```python
from build123d import *

# Parameters (mm, degrees)
BOSS_EXTRUDE1_DEPTH = 10
BOSS_EXTRUDE2_DEPTH = 10
MIRROR1_START       = 20
MIRROR1_DEPTH       = 20
MIRROR1_START_2     = 30
MIRROR1_2_DEPTH     = 10
MIRROR1_3_DEPTH     = 10
FILLET1_R           = 2
FILLET2_R           = 1
SKETCH3_R           = 11
BOSS_EXTRUDE3_DEPTH = 2
SKETCH4_R           = 1.5
CUT_EXTRUDE1_DEPTH  = 4.5
SKETCH5_R           = 2.5
CUT_EXTRUDE3_DEPTH  = 52.521063654
CHAMFER3_SIZE       = 0.4
BOSS_EXTRUDE4_START = -59
SKETCH6_R           = 2.5
BOSS_EXTRUDE4_DEPTH = 59
CUT_EXTRUDE8_DEPTH  = 17


# Read off the part's stored shape, not the designer's step: Mirror1
with BuildPart() as part:
    # Sketch1 → Boss-Extrude1 (new body)
    with BuildSketch(Plane(origin=(0, 0, 0), x_dir=(1, 0, 0), z_dir=(0, 1, 0))):
        Polygon((-21, 16), (-16, 21), (16, 21), (21, 16), (21, -16), (16, -21), (-16, -21), (-21, -16), align=None)
    extrude(amount=BOSS_EXTRUDE1_DEPTH)

    # Sketch2 → Boss-Extrude2 (add)
    with BuildSketch(Plane(origin=(0, 10, 0), x_dir=(1, 0, 0), z_dir=(0, 1, 0))):
        Polygon((-21.1, 11.1), (-11.1, 21.1), (11.1, 21.1), (21.1, 11.1), (21.1, -11.1), (11.1, -21.1), (-11.1, -21.1), (-21.1, -11.1), align=None)
    extrude(amount=BOSS_EXTRUDE2_DEPTH)

    # Mirror1 outline → Mirror1 (add)
    with BuildSketch(Plane(origin=(0, 0, 0), x_dir=(1, 0, 0), z_dir=(0, 1, 0)).offset(MIRROR1_START)):
        Polygon((-21, 11.2), (-21, -11.2), (-11.2, -21), (11.2, -21), (21, -11.2), (21, 11.2), (11.2, 21), (-11.2, 21), align=None)
    extrude(amount=MIRROR1_DEPTH)

    # Mirror1 2 outline → Mirror1 2 (add)
    with BuildSketch(Plane(origin=(0, 0, 0), x_dir=(1, 0, 0), z_dir=(0, 1, 0)).offset(MIRROR1_START_2)):
        Polygon((-21, -11.2), (-21, -16), (-16, -21), (-11.2, -21), align=None)
        Polygon((-21, 16), (-21, 11.2), (-11.2, 21), (-16, 21), align=None)
        Polygon((21, -11.2), (11.2, -21), (16, -21), (21, -16), align=None)
        Polygon((16, 21), (11.2, 21), (21, 11.2), (21, 16), align=None)
    extrude(amount=MIRROR1_2_DEPTH)

    # Mirror1 3 outline → Mirror1 3 (add)
    with BuildSketch(Plane(origin=(0, 0, 0), x_dir=(1, 0, 0), z_dir=(0, 1, 0)).offset(MIRROR1_START)):
        Polygon((-21.1, -11.1), (-21, -11.2), (-21, 11.2), (-21.1, 11.1), align=None)
        Polygon((11.2, -21), (-11.2, -21), (-11.1, -21.1), (11.1, -21.1), align=None)
        Polygon((-11.1, 21.1), (-11.2, 21), (11.2, 21), (11.1, 21.1), align=None)
        Polygon((21, 11.2), (21, -11.2), (21.1, -11.1), (21.1, 11.1), align=None)
    extrude(amount=MIRROR1_3_DEPTH)

    # Fillet1
    # the kernel refuses this fillet: 2 mm, written as the material it takes off along each edge
    with BuildSketch(Plane(origin=(11.1, 10, -21.1), x_dir=(0.7071067811865497, 0, 0.7071067811865454), z_dir=(0, 1, 0)), Plane(origin=(-11.1, 30, -21.1), x_dir=(-0.707106781186553, 0, 0.7071067811865422), z_dir=(0, -1, 0)), Plane(origin=(-21.1, 10, -11.1), x_dir=(0.7071067811865487, 0, -0.7071067811865465), z_dir=(0, 1, 0)), Plane(origin=(-21.1, 30, 11.1), x_dir=(0.7071067811865239, 1.1932702685997172e-15, 0.7071067811865711), z_dir=(0, -1, 0)), Plane(origin=(-11.1, 10, 21.1), x_dir=(-0.7071067811865497, 0, -0.7071067811865454), z_dir=(0, 1, 0)), Plane(origin=(21.1, 30, -11.1), x_dir=(-0.7071067811865326, 1.3816813636417406e-15, -0.7071067811865626), z_dir=(0, -1, 0))) as fillet1_piece_1:
        with BuildLine():
            CenterArc((FILLET1_R * 0.414213562373, -FILLET1_R), FILLET1_R, 90, 45)
            Line((-FILLET1_R * 0.292893218813, -FILLET1_R * 0.292893218813), (0, 0))
            Line((0, 0), (FILLET1_R * 0.414213562373, 0))
        make_face()
    extrude(amount=20, mode=Mode.SUBTRACT)
    with BuildSketch(Plane(origin=(11.1, 10, 21.1), x_dir=(0.7071067811865465, 0, -0.7071067811865487), z_dir=(0, 1, 0)), Plane(origin=(21.1, 30, 11.1), x_dir=(-0.7071067811865475, 0, 0.7071067811865475), z_dir=(0, -1, 0))) as fillet1_piece_2:
        with BuildLine():
            CenterArc((FILLET1_R * 0.414213562373, FILLET1_R), FILLET1_R, 225, 45)
            Line((-FILLET1_R * 0.292893218813, FILLET1_R * 0.292893218813), (0, 0))
            Line((0, 0), (FILLET1_R * 0.414213562373, 0))
        make_face()
    extrude(amount=20, mode=Mode.SUBTRACT)

    # Fillet2
    fillet2_edges = [part.edges().sort_by_distance(p)[0] for p in [
        (-21, 5, -16),
        (-16, 5, -21),
        (16, 5, -21),
        (21, 5, -16),
        (21, 5, 16),
        (16, 5, 21),
        (-16, 5, 21),
        (-21, 5, 16),
        (-21, 35, 16),
        (-16, 35, 21),
        (16, 35, 21),
        (21, 35, 16),
        (21, 35, -16),
        (16, 35, -21),
        (-16, 35, -21),
        (-21, 35, -16),
    ]]
    fillet(fillet2_edges, radius=FILLET2_R)

    # Sketch3 → Boss-Extrude3 (add)
    with BuildSketch(Plane(origin=(0, 40, 0), x_dir=(1, 0, 0), z_dir=(0, 1, 0))):
        with Locations(Location((0, 0, 0), (0, 0, 270))):
            Circle(SKETCH3_R)
    extrude(amount=BOSS_EXTRUDE3_DEPTH)

    # Sketch4 → Cut-Extrude1 (cut)
    with BuildSketch(Plane(origin=(0, 40, 0), x_dir=(1, 0, 0), z_dir=(0, 1, 0))):
        with Locations(Location((-15.5, 15.5, 0), (0, 0, 270))):
            Circle(SKETCH4_R)
        with Locations(Location((15.5, 15.5, 0), (0, 0, 270))):
            Circle(SKETCH4_R)
        with Locations(Location((15.5, -15.5, 0), (0, 0, 270))):
            Circle(SKETCH4_R)
        with Locations(Location((-15.5, -15.5, 0), (0, 0, 270))):
            Circle(SKETCH4_R)
    extrude(amount=-CUT_EXTRUDE1_DEPTH, mode=Mode.SUBTRACT)

    # Sketch5 → Cut-Extrude3 (cut, through all)
    with BuildSketch(Plane(origin=(0, 42, 0), x_dir=(1, 0, 0), z_dir=(0, 1, 0))):
        with Locations(Location((0, 0, 0), (0, 0, 270))):
            Circle(SKETCH5_R)
    extrude(amount=-CUT_EXTRUDE3_DEPTH, mode=Mode.SUBTRACT)

    # Chamfer3
    chamfer3_edges = [part.edges().sort_by_distance(p)[0] for p in [
        (0, 42, -2.5),
    ]]
    chamfer(chamfer3_edges, length=CHAMFER3_SIZE)

    # Sketch6 → Boss-Extrude4 (add)
    with BuildSketch(Plane.XZ.offset(BOSS_EXTRUDE4_START)):
        with Locations(Location((0, 0, 0), (0, 0, 90))):
            Circle(SKETCH6_R)
    extrude(amount=BOSS_EXTRUDE4_DEPTH)

    # Sketch7 → Cut-Extrude8 (cut)
    with BuildSketch(Plane(origin=(0, 59, 0), x_dir=(1, 0, 0), z_dir=(0, 1, 0))):
        with BuildLine():
            Line((1.947589111, 1.567449092), (-1.709469516, 1.824202284))
            ThreePointArc((-1.709469516, 1.824202284), (0.175087938, 2.493861306), (1.947589111, 1.567449092))
        make_face()
    extrude(amount=-CUT_EXTRUDE8_DEPTH, mode=Mode.SUBTRACT)


solid = part.part
```
Design review of the part built by this model. Coordinates are the model's own, in mm. A direction names the side the tool comes from. Coordinates: 2 decimals unless noted, no trailing zeros. Order: outer loops, then holes, each group sorted by start corner. A loop starts at its lowest first (then second) coordinate and runs counter-clockwise, first axis right, second up. Notation, with made-up numbers: (84.5, 42.5) - (89.5, 42.5) arc R20 cw to (89.5, 76.5) - close; hole circle Ø8 at (78.25, 9.25). An arc over 180 degrees is marked (long way). One line per question, with ' | ' between items.
Q1. Consider section D-D, the plane x = 0. Give the boundary of the cut face in (y, z).
Answer key:
outline: (0, -21) - (10, -21) - (10, -21.1) - (30, -21.1) - (30, -21) - (40, -21) - (40, -11) - (42, -11) - (42, -2.9) - (41.6, -2.5) - (42, -2.5) - (42, -1.7) - (59, -1.7) - (59, 2.5) - (41.6, 2.5) - (42, 2.9) - (42, 11) - (40, 11) - (40, 21) - (30, 21) - (30, 21.1) - (10, 21.1) - (10, 21) - (0, 21) - close
Q2. The part is to be moulded in two halves that separate along Y. For faces 4 (the flat face through (-16.2, 19.9, 16)), 5 (the flat face through (-17, 10, -17)), 6 (the flat face through (-2.3, 42, 2.3)), 7 (the flat face through (0, 5, -21)), say which applies: +Y half, -Y half, draft (parallel to the pull), parting line (faces both ways), or undercut.
Answer key:
face 4: undercut | face 5: undercut | face 6: +Y half | face 7: draft
Q3. To check wall thickness, follow line 1 along X through (y, z) = (38.85, 15.5); line 2 along X through (y, z) = (36, 15); line 3 along Y through (x, z) = (2, 12). State the ranges of each line that lie inside material, in increasing order.
Answer key:
line 1: x = -21 to -17, -14 to 14, 17 to 21 | line 2: x = -21 to -16.91, -14.09 to 14.09, 16.91 to 21 | line 3: y = 0 to 40
Q4. Consider section C-C, the plane x = 5. Give the boundary of the cut face in (y, z).
Answer key:
outline: (0, -21) - (10, -21) - (10, -21.1) - (30, -21.1) - (30, -21) - (40, -21) - (40, -9.8) - (42, -9.8) - (42, 9.8) - (40, 9.8) - (40, 21) - (30, 21) - (30, 21.1) - (10, 21.1) - (10, 21) - (0, 21) - close
Q5. Clearance check with flat-ended pins moving along their axes: pin 1 Ø1 at (y, z) = (42, 15.5) entering from -X; pin 2 Ø8 at (x, z) = (18, 16.5) entering from -Y; pin 3 Ø1.5 at (x, z) = (15, -8) entering from +Y; pin 4 Ø8 at (y, z) = (35.5, 6.5) entering from +X. State where each tip first meets the part, or that it passes through.
Answer key:
pin 1: passes through | pin 2: stops at y = 0 | pin 3: stops at y = 40 | pin 4: stops at x = 21
Q6. Consider section B-B, the plane z = 0. Give the boundary of the cut face in (x, y).
Answer key:
outline: (-21.1, 10) - (-21, 10) - (-21, 0) - (21, 0) - (21, 10) - (21.1, 10) - (21.1, 30) - (21, 30) - (21, 40) - (11, 40) - (11, 42) - (2.9, 42) - (2.5, 41.6) - (2.5, 59) - (-2.5, 59) - (-2.5, 41.6) - (-2.9, 42) - (-11, 42) - (-11, 40) - (-21, 40) - (-21, 30) - (-21.1, 30) - close
Q7. For faces 1 (the flat face through (-16, 19.9, -16.2)), 2 (the flat face through (0.145, 50.619, -1.694)), 3 (the flat face through (-21, 5, 0)), list the 3-axis set-ups (+Z, -Z, +X, -X, +Y, -Y) from which the entire face can be reached by the end or side of a thin tool; tool diameter is ignored.
Answer key:
face 1: -Z, -X | face 2: -Z, +X, +Y | face 3: +Z, -Z, -X, -Y
Q8. Consider section A-A, the plane y = 9. Give the boundary of the cut face in (x, z), then the cut area to 3 significant figures.
Answer key:
outline: (-21, -15.59) arc R1 ccw to (-20.71, -16.29) - (-16.29, -20.71) arc R1 ccw to (-15.59, -21) - (15.59, -21) arc R1 ccw to (16.29, -20.71) - (20.71, -16.29) arc R1 ccw to (21, -15.59) - (21, 15.59) arc R1 ccw to (20.71, 16.29) - (16.29, 20.71) arc R1 ccw to (15.59, 21) - (-15.59, 21) arc R1 ccw to (-16.29, 20.71) - (-20.71, 16.29) arc R1 ccw to (-21, 15.59) - close | area: 1,710 mm2
